Can you work these out from the model? Positions are in its coordinate system, mm. A direction names the side the tool comes from. Round coordinates to 2 decimals unless told otherwise and drop trailing zeros. Order: outer loops, then holes, each group sorted by start corner. A loop starts at its lowest first (then second) coordinate and runs counter-clockwise, first axis right, second up.
from build123d import *

# Parameters (mm, degrees)
F0_R     = 11
F1_DEPTH = 7


# Not quite as in the source:
# - a feature of the source that left no trace in its solid (it failed there, or was rolled back) is left out


with BuildPart() as f1:
    # F0 (on Top) → F1 (new body)
    with BuildSketch(Plane.XY):
        with BuildLine():
            ThreePointArc((-33.6919065778, -12.4136305481), (-22.2121981946, -14.8954900703), (-12.4070507332, -8.4300113941))
            ThreePointArc((-12.4070507332, -8.4300113941), (-9.2272824926, -11.8261260691), (-5.1598693222, -14.0845925954))
            Line((-5.1598693222, -14.0845925954), (0, -15.0684863329))
            Line((0, -15.0684863329), (4.9237644598, -14.1688582301))
            ThreePointArc((4.9237644598, -14.1688582301), (9.1941581889, -11.851896692), (12.5, -8.2915619759))
            ThreePointArc((12.5, -8.2915619759), (22.2312035836, -14.7988434658), (33.6847114379, -12.378472956))
            add(Edge.make_bspline(
                [(36.6861147035, -9.6232201138), (35.4322184653, -9.3782649416), (32.9856759013, -8.9056095075), (33.4504308992, -11.233519818), (33.6847114379, -12.378472956)],
                knots=[0.0023635799, 0.0023635799, 0.0023635799, 0.0023635799, 0.5096931431, 0.9950324973, 0.9950324973, 0.9950324973, 0.9950324973], degree=3))
            ThreePointArc((36.6861147035, -9.6232201138), (38.2829241904, -7.281044503), (39.4129405486, -4.6813041007))
            add(Edge.make_bspline(
                [(39.3532489974, 4.8612453714), (40.0640178656, 3.2496024167), (40.675386779, 0.0090485332), (40.094980448, -3.1441618112), (39.4129405486, -4.6813041007)],
                knots=[0, 0, 0, 0, 0.5048307155, 1, 1, 1, 1], degree=3))
            ThreePointArc((39.3532489974, 4.8612453714), (38.2366644679, 7.3653393625), (36.6849282767, 9.6257292672))
            add(Edge.make_bspline(
                [(33.6844640266, 12.3797240959), (33.4791642411, 11.4442056961), (33.0552816759, 9.4534774659), (35.4207112642, 9.5639432605), (36.6849282767, 9.6257292672)],
                knots=[0.0055976008, 0.0055976008, 0.0055976008, 0.0055976008, 0.4689523637, 0.9973928627, 0.9973928627, 0.9973928627, 0.9973928627], degree=3))
            ThreePointArc((33.6844640266, 12.3797240959), (22.2307373346, 14.7998328025), (12.4996432587, 8.2920997584))
            ThreePointArc((12.4996432587, 8.2920997584), (9.1939032334, 11.8520944704), (4.9237644598, 14.1688582301))
            Line((4.9237644598, 14.1688582301), (0, 15.0684863329))
            Line((0, 15.0684863329), (-5.1598693222, 14.0845925954))
            ThreePointArc((-5.1598693222, 14.0845925954), (-9.2272824926, 11.8261260691), (-12.4070507332, 8.4300113941))
            ThreePointArc((-12.4070507332, 8.4300113941), (-22.2121981946, 14.8954900703), (-33.6919065778, 12.4136305481))
            Line((-33.6919065778, 12.4136305481), (-37.2543297708, 17.1683672816))
            Line((-37.2543297708, 17.1683672816), (-40.6296290457, 12.4136305481))
            Line((-40.6296290457, 12.4136305481), (-36.703640056, 9.6266439002))
            ThreePointArc((-36.703640056, 9.6266439002), (-38.2445317988, 7.3640913066), (-39.3532489974, 4.8612453714))
            add(Edge.make_bspline(
                [(-39.3532489974, 4.8612453714), (-40.2528289587, 3.2490634103), (-40.4878486023, 0.0095823751), (-40.2812252759, -3.1446904889), (-39.4129405486, -4.6813041007)],
                knots=[0, 0, 0, 0, 0.5048307155, 1, 1, 1, 1], degree=3))
            ThreePointArc((-39.4129405486, -4.6813041007), (-38.2903364161, -7.2811002801), (-36.703640056, -9.6266439002))
            Line((-36.703640056, -9.6266439002), (-40.6296290457, -12.4136305481))
            Line((-40.6296290457, -12.4136305481), (-37.2543297708, -17.1683672816))
            Line((-37.2543297708, -17.1683672816), (-33.6919065778, -12.4136305481))
        make_face()
        with Locations((-25, 0)):
            Circle(F0_R, mode=Mode.SUBTRACT)
        with BuildLine():
            ThreePointArc((0, -11), (-11, 0), (0, 11))
            ThreePointArc((0, 11), (11, 0), (0, -11))
        make_face(mode=Mode.SUBTRACT)
        with Locations((25, 0)):
            Circle(F0_R, mode=Mode.SUBTRACT)
        with BuildLine():
            ThreePointArc((33.8754488345, -12.2437849019), (33.7803409626, -12.3114982961), (33.6847114379, -12.378472956))
            add(Edge.make_bspline(
                [(33.6847114379, -12.378472956), (33.6871093254, -12.3901916797), (33.6895079516, -12.4019111139), (33.6919065778, -12.4136305481)],
                knots=[0.9950324973, 0.9950324973, 0.9950324973, 0.9950324973, 1, 1, 1, 1], degree=3))
            Line((33.6919065778, -12.4136305481), (33.8754488345, -12.2437849019))
        make_face()
        with BuildLine():
            add(Edge.make_bspline(
                [(36.6861147035, -9.6232201138), (35.4322184653, -9.3782649416), (32.9856759013, -8.9056095075), (33.4504308992, -11.233519818), (33.6847114379, -12.378472956)],
                knots=[0.0023635799, 0.0023635799, 0.0023635799, 0.0023635799, 0.5096931431, 0.9950324973, 0.9950324973, 0.9950324973, 0.9950324973], degree=3))
            ThreePointArc((33.6847114379, -12.378472956), (33.7803409626, -12.3114982961), (33.8754488345, -12.2437849019))
            Line((33.8754488345, -12.2437849019), (33.6919065778, -12.4136305481))
            Line((33.6919065778, -12.4136305481), (37.2543297708, -17.1683672816))
            Line((37.2543297708, -17.1683672816), (40.6296290457, -12.4136305481))
            Line((40.6296290457, -12.4136305481), (36.703640056, -9.6266439002))
            Line((36.703640056, -9.6266439002), (36.6135832636, -9.7099803175))
            ThreePointArc((36.6135832636, -9.7099803175), (36.6499303523, -9.6666682398), (36.6861147035, -9.6232201138))
        make_face()
        with BuildLine():
            add(Edge.make_bspline(
                [(36.703640056, -9.6266439002), (36.6977982463, -9.6255026135), (36.6919564367, -9.6243613269), (36.6861147035, -9.6232201138)],
                knots=[0, 0, 0, 0, 0.0023635799, 0.0023635799, 0.0023635799, 0.0023635799], degree=3))
            ThreePointArc((36.6861147035, -9.6232201138), (36.6499303523, -9.6666682398), (36.6135832636, -9.7099803175))
            Line((36.6135832636, -9.7099803175), (36.703640056, -9.6266439002))
        make_face()
        with BuildLine():
            ThreePointArc((36.6176990871, 9.7061716321), (36.6513836228, 9.6660089023), (36.6849282767, 9.6257292672))
            add(Edge.make_bspline(
                [(36.6849282767, 9.6257292672), (36.6911654734, 9.6260340973), (36.6974027647, 9.6263389988), (36.703640056, 9.6266439002)],
                knots=[0.9973928627, 0.9973928627, 0.9973928627, 0.9973928627, 1, 1, 1, 1], degree=3))
            Line((36.703640056, 9.6266439002), (36.6176990871, 9.7061716321))
        make_face()
        with BuildLine():
            add(Edge.make_bspline(
                [(33.6844640266, 12.3797240959), (33.4791642411, 11.4442056961), (33.0552816759, 9.4534774659), (35.4207112642, 9.5639432605), (36.6849282767, 9.6257292672)],
                knots=[0.0055976008, 0.0055976008, 0.0055976008, 0.0055976008, 0.4689523637, 0.9973928627, 0.9973928627, 0.9973928627, 0.9973928627], degree=3))
            ThreePointArc((36.6849282767, 9.6257292672), (36.6513836228, 9.6660089023), (36.6176990871, 9.7061716321))
            Line((36.6176990871, 9.7061716321), (36.703640056, 9.6266439002))
            Line((36.703640056, 9.6266439002), (40.6296290457, 12.4136305481))
            Line((40.6296290457, 12.4136305481), (37.2543297708, 17.1683672816))
            Line((37.2543297708, 17.1683672816), (33.6919065778, 12.4136305481))
            Line((33.6919065778, 12.4136305481), (33.8702569567, 12.2485893424))
            ThreePointArc((33.8702569567, 12.2485893424), (33.777607815, 12.3145071292), (33.6844640266, 12.3797240959))
        make_face()
        with BuildLine():
            add(Edge.make_bspline(
                [(33.6919065778, 12.4136305481), (33.6894253739, 12.4023281311), (33.68694417, 12.391025714), (33.6844640266, 12.3797240959)],
                knots=[0, 0, 0, 0, 0.0055976008, 0.0055976008, 0.0055976008, 0.0055976008], degree=3))
            ThreePointArc((33.6844640266, 12.3797240959), (33.777607815, 12.3145071292), (33.8702569567, 12.2485893424))
            Line((33.8702569567, 12.2485893424), (33.6919065778, 12.4136305481))
        make_face()
    extrude(amount=F1_DEPTH)


solid = f1.part
(1) I want a section at A-A, the plane x = -25. List the corners of the cut face in (y, z) for me.
(2) I'm going to push flat-ended pins straight in: pin 1 Ø3 at (x, z) = (-3.5, 5.5) entering from +Y; pin 2 Ø1 at (x, z) = (-0.5, 5.5) entering from -Y; pin 3 Ø10 at (x, y) = (9.5, -5.5) entering from +Z; pin 4 Ø13 at (x, y) = (0, 0) entering from -Z. Where does each tip first touch, or does it pass through?
(3) If we mould it in two halves opening along X, with no side actions, what happens to faces 1 (the face through (-38.309, -7.246, 3.451)), 2 (the face through (-14.839, -4.213, 3.451)), 3 (the face through (38.64, 11, 3.45))? For each: pulls with the +X half, pulls with the -X half, needs draft (parallel to the pull), parting line crosses it, or undercut.
(4) I want a section at D-D, the plane x = 3.5. List the corners of the cut face in (y, z) for me, plus the area to 3 significant figures.
(5) Please list where these lines run through material, in increasing order: probe 1 along Y at (x, z) = (-25, 3); probe 2 along X at (y, z) = (8, 6); probe 3 along X at (y, z) = (-2.5, 5).
(6) I want a section at B-B, the plane y = 7.5. List the corners of the cut face in (x, z) for me.
(7) I want a section at C-C, the plane z = 3.75. Give the number of separate pieces and of enclosed holes in the cut face, plus the area to 3 significant figures.
(8) On a 3-axis mill with a long thin cutter (end or side, diameter ignored), from which of +Z, -Z, +X, -X, +Y, -Y can I reach the whole of each face in a straight line? I mean faces 4 (the face through (38.694, -11.04, 3.451)), 5 (the face through (-38.694, 11.04, 3.451)), 6 (the face through (35.161, -4.213, 3.451)), 7 (the face through (-2.62, -14.57, 3.45)), 8 (the face through (2.5, 14.61, 3.45)). Say none if no direction works.
Ans:
1. outline: (-15.15, 0) - (-11, 0) - (-11, 7) - (-15.15, 7) - close; (11, 0) - (15.15, 0) - (15.15, 7) - (11, 7) - close
2. pin 1: stops at y = 14.69
2. pin 2: stops at y = -15.07
2. pin 3: stops at z = 7
2. pin 4: passes through
3. face 1: pulls with the -X half
3. face 2: undercut
3. face 3: pulls with the +X half
4. outline: (-14.43, 0) - (-10.43, 0) - (-10.43, 7) - (-14.43, 7) - close; (10.43, 0) - (14.43, 0) - (14.43, 7) - (10.43, 7) - close
4. area: 56.0 mm2
5. probe 1: y = -15.15 to -11, 11 to 15.15
5. probe 2: x = -37.87 to -32.55, -17.45 to -7.55, 7.55 to 17.45, 32.55 to 37.86
5. probe 3: x = -40.2 to -35.71, -14.29 to -10.71, 10.71 to 14.29, 35.71 to 40.12
6. outline: (-38.17, 0) - (-33.05, 0) - (-33.05, 7) - (-38.17, 7) - close; (-16.95, 0) - (-8.05, 0) - (-8.05, 7) - (-16.95, 7) - close; (8.05, 0) - (16.95, 0) - (16.95, 7) - (8.05, 7) - close; (33.05, 0) - (38.16, 0) - (38.16, 7) - (33.05, 7) - close
7. separate pieces: 1
7. enclosed holes: 3
7. area: 991 mm2
8. face 4: +Z, -Z, +X
8. face 5: +Z, -Z, -X
8. face 6: +Z, -Z
8. face 7: +Z, -Z, -Y
8. face 8: +Z, -Z, +Y
